from build123d import *

# Parameters (mm, degrees)
F0_W           = 306.5
F0_H           = 110
F1_DEPTH       = 13
F2_D           = 9
F2_CSINK_D     = 11.2
F2_CSINK_ANGLE = 90
F3_D           = 80
F4_D           = 10.3


with BuildPart() as f1:
    # F0 (on Top) → F1 (new body)
    with BuildSketch(Plane.XY):
        Rectangle(F0_W, F0_H)
    extrude(amount=F1_DEPTH)

    # F2 (through all)
    with Locations(Plane(origin=(0, 0, 0), x_dir=(1, 0, 0), z_dir=(0, 0, -1))):
        with Locations((-113.25, 0), (-63.25, 0), (76.75, 0), (126.75, 0)):
            CounterSinkHole(F2_D / 2, F2_CSINK_D / 2, counter_sink_angle=F2_CSINK_ANGLE)

    # F3 (through all)
    with Locations(Plane(origin=(0, 0, 0), x_dir=(1, 0, 0), z_dir=(0, 0, -1))):
        with Locations((6.75, 0)):
            Hole(F3_D / 2)

    # F4 (through all)
    with Locations(Plane(origin=(0, 0, 0), x_dir=(1, 0, 0), z_dir=(0, 0, -1))):
        with Locations((-133.25, 40), (-78.25, 40), (-133.25, -40), (-78.25, -40), (91.75, 40), (136.75, 40), (91.75, -40), (136.75, -40)):
            Hole(F4_D / 2)


solid = f1.part
Geometry: final body of the model. Coordinates: model frame, mm. Coordinates: 2 decimals unless noted, no trailing zeros. Loops run counter-clockwise (first coordinate to the right, second up) from the corner with the lowest first, then second, coordinate; pieces in that order, holes last. Notation, with made-up numbers: (35.5, -13.75) - (93.5, -13.75) arc R32 ccw to (93.5, 19.25) - close; hole circle Ø2 at (-3.5, 25). An arc over 180 degrees is marked (long way). One line per question, with ' | ' between items. Start each with the question number.
(1) Cut plane D-D on x = 6.75. Output: boundary loops of the cut face in (y, z), and give its area (3 significant figures).
(2) Cut plane C-C on x = 136.75. Output: boundary loops of the cut face in (y, z), and give its area (3 significant figures).
(3) Draft query along Y for faces 1 (the cylindrical face through (86.84, 38.45, 6.59)), 2 (the cylindrical face through (-83.16, 38.45, 6.59)), 3 (the flat face through (-36, 1, 0)). Return one class per face: +Y half, -Y half, draft (parallel to the pull), parting line (faces both ways), or undercut.
(4) Ray query, L1, parallel to Y at x = 91.75, z = 7; L2, parallel to Y at x = -63.25, z = 9.5; L3, parallel to X at y = 4, z = 11. Return the intervals inside material, ascending. Write a range as from..to.
(5) Cut plane A-A on z = 3.5. Count the separate pieces of the cut face and the enclosed holes in it, and give its area (3 significant figures).
(6) Cut plane B-B on x = 76.75. Output: boundary loops of the cut face in (y, z).
Here are the results:
1) outline: (-55, 0) - (-40, 0) - (-40, 13) - (-55, 13) - close; (40, 0) - (55, 0) - (55, 13) - (40, 13) - close | area: 390 mm²
2) outline: (-55, 0) - (-45.15, 0) - (-45.15, 13) - (-55, 13) - close; (-34.85, 0) - (34.85, 0) - (34.85, 13) - (-34.85, 13) - close; (45.15, 0) - (55, 0) - (55, 13) - (45.15, 13) - close | area: 1,160 mm²
3) face 1: undercut | face 2: undercut | face 3: draft
4) L1: -55..-45.15, -34.85..34.85, 45.15..55 | L2: -55..-4.5, 4.5..55 | L3: -153.25..-115.31, -111.19..-65.31, -61.19..-33.05, 46.55..74.69, 78.81..124.69, 128.81..153.25
5) separate pieces: 1 | enclosed holes: 13 | area: 27,800 mm²
6) outline: (-55, 0) - (-5.6, 0) - (-4.5, 1.1) - (-4.5, 13) - (-55, 13) - close; (4.5, 1.1) - (5.6, 0) - (55, 0) - (55, 13) - (4.5, 13) - close
